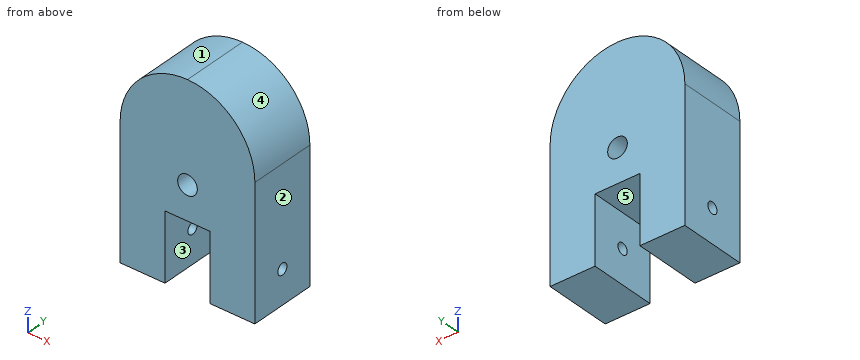
```python
from build123d import *

# Parameters (mm, degrees)
F1_DEPTH = 76.2
F2_R     = 76.19999
F4_D     = 22.225
F6_D     = 12.7


# Not quite as in the source:
# - a fillet or chamfer is up to 0.001 mm smaller than in the source, because OpenCascade refuses the exact size


with BuildPart() as f1:
    # F0 (on Front) → F1 (new body)
    with BuildSketch(Plane.XZ):
        Polygon((-50.8, 0), (0, 0), (0, 76.2), (50.8, 76.2), (50.8, 0), (101.6, 0), (101.6, 225.425), (-50.8, 225.425), align=None)
    extrude(amount=F1_DEPTH)

    # F2 (radius 76.2 in the source; OpenCascade refuses exactly that, so slightly less here)
    f2_edges = [f1.edges().sort_by_distance(p)[0] for p in [
        (101.6, -38.1, 225.425),
        (-50.8, -38.1, 225.425),
    ]]
    fillet(f2_edges, radius=F2_R)

    # F4 (through all)
    with Locations(Plane.XZ.offset(76.2)):
        with Locations((25.4, 114.3)):
            Hole(F4_D / 2)

    # F6 (through all)
    with Locations(Plane.YZ.offset(101.6)):
        with Locations((-38.1, 38.1)):
            Hole(F6_D / 2)


solid = f1.part
```
Model file for the job. Use its own axes, mm. Face numbers are marked on the shaded views. A direction names the side the tool comes from. Coordinates: 2 decimals unless noted, no trailing zeros. Loops run counter-clockwise (first coordinate to the right, second up) from the corner with the lowest first, then second, coordinate; pieces in that order, holes last. Notation, with made-up numbers: (72.5, 49.25) - (123.5, 49.25) arc R27 ccw to (123.5, 67.25) - close; hole circle Ø7 at (31.5, 57). An arc over 180 degrees is marked (long way). Answer as a JSON object with one key per item and string values. Group by question number.
(1) Two-plate mould, pull along X, no slides. Class the marked faces 1, 2 and 3: released by +X, released by -X, zero draft, split by the parting line, or undercut.
(2) Flat gauge pins, fed straight in: pin 1 (1.5 mm diameter, centred on x = 42, y = -26, fed in from -Z); pin 2 (2 mm diameter, centred on x = 39.5, y = -44.5, fed in from +Z); pin 3 (1.5 mm diameter, centred on x = -14, y = -52.5, fed in from +Z). Where does each tip first touch, or does it go through?
(3) Tool access for the marked faces 4 and 5: list every direction of +Z, -Z, +X, -X, +Y, -Y with a clear straight run to the whole face (end or side of a thin tool).
(4) Probe line 1 along X through (y, z) = (-71.5, 38); line 2 along X through (y, z) = (-54, 114); line 3 along Y through (x, z) = (-12, 38). List the from-to ranges inside material, lowest first.
(5) Cut at A-A (z = 19.5). Give the cut face in (x, y).
(6) Cut at B-B (y = -38.1). State how many separate pieces and enclosed holes the cut face has, then the cut area to 3 significant figures.
(7) Cut at D-D (x = 18). Give the cut face in (y, z), then the cut area to 3 significant figures.
Geometry says:
{
 "1": {"face 1": "released by -X", "face 2": "released by +X", "face 3": "undercut"},
 "2": {"pin 1": "stops at z = 76.2", "pin 2": "stops at z = 224.29", "pin 3": "stops at z = 214.9"},
 "3": {"face 4": "+Z, +X, +Y, -Y", "face 5": "-Z, +Y, -Y"},
 "4": {"line 1": "x = -50.8 to 0, 50.8 to 101.6", "line 2": "x = -50.8 to 14.29, 36.51 to 101.6", "line 3": "y = -76.2 to -44.45, -31.75 to 0"},
 "5": {"outline": "(-50.8, -76.2) - (0, -76.2) - (0, 0) - (-50.8, 0) - close; (50.8, -76.2) - (101.6, -76.2) - (101.6, 0) - (50.8, 0) - close"},
 "6": {"separate pieces": "3", "enclosed holes": "1", "area": "26,300 mm^2"},
 "7": {"outline": "(-76.2, 76.2) - (0, 76.2) - (0, 106.01) - (-76.2, 106.01) - close; (-76.2, 122.59) - (0, 122.59) - (0, 225.06) - (-76.2, 225.06) - close", "area": "10,100 mm^2"}
}
